from build123d import *

# Parameters (mm, degrees)
SKETCH1_W           = 100
SKETCH1_H           = 100
SKETCH1_W_2         = 96
SKETCH1_H_2         = 96
EXTRUDE_THIN1_DEPTH = 10
FILLET1_R           = 5
FILLET2_R           = 3
BOSS_EXTRUDE1_DEPTH = 1


with BuildPart() as part:
    # Sketch1 → Extrude-Thin1 (new body)
    with BuildSketch(Plane(origin=(0, 0, 0), x_dir=(1, 0, 0), z_dir=(0, 1, 0))):
        Rectangle(SKETCH1_W, SKETCH1_H)
        Rectangle(SKETCH1_W_2, SKETCH1_H_2, mode=Mode.SUBTRACT)
    extrude(amount=EXTRUDE_THIN1_DEPTH)

    # Fillet1
    fillet1_edges = [part.edges().sort_by_distance(p)[0] for p in [
        (50, 5, 50),
        (-50, 5, 50),
        (-50, 5, -50),
        (50, 5, -50),
    ]]
    fillet(fillet1_edges, radius=FILLET1_R)

    # Fillet2
    fillet2_edges = [part.edges().sort_by_distance(p)[0] for p in [
        (48, 5, 48),
        (48, 5, -48),
        (-48, 5, -48),
        (-48, 5, 48),
    ]]
    fillet(fillet2_edges, radius=FILLET2_R)

    # Sketch2 → Boss-Extrude1 (add)
    with BuildSketch(Plane.XZ):
        with BuildLine():
            Line((45, 50), (-45, 50))
            ThreePointArc((-45, 50), (-48.535533906, 48.535533906), (-50, 45))
            Line((-50, 45), (-50, -45))
            ThreePointArc((-50, -45), (-48.535533906, -48.535533906), (-45, -50))
            Line((-45, -50), (45, -50))
            ThreePointArc((45, -50), (48.535533906, -48.535533906), (50, -45))
            Line((50, -45), (50, 45))
            ThreePointArc((50, 45), (48.535533906, 48.535533906), (45, 50))
        make_face()
    extrude(amount=BOSS_EXTRUDE1_DEPTH)


solid = part.part
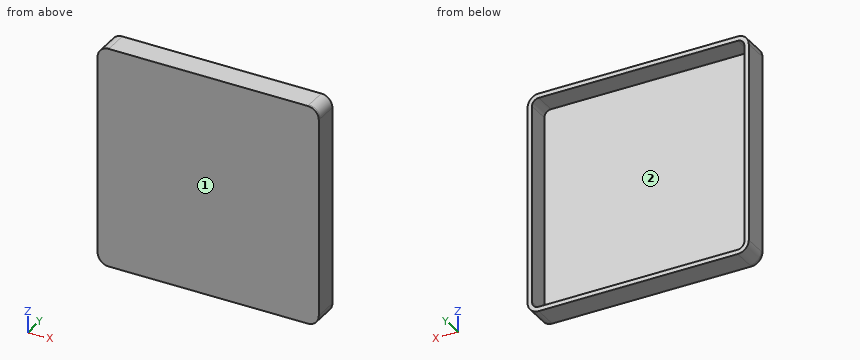
Here's how the part is built. I have some questions about the finished solid (model axes, mm). Face numbers are marked on the shaded views. Coordinates: 2 decimals unless noted, no trailing zeros. Write each loop counter-clockwise with the first axis right and the second up, starting at its lowest first coordinate (ties: lowest second). Pieces come first, ordered by that corner, then holes.
Item 1: If I drill on line 1 (Z direction, x = -40.5, y = 2.25); line 2 (Y direction, x = -7.5, z = -3), over which ranges is the centre line in solid material (lowest first)?
Item 2: I want a section at B-B on x = 34. Write out the boundary of the cut face in (y, z).
Item 3: If we mould it in two halves opening along Z, with no side actions, what happens to the marked faces 1 and 2? For each: +Z half, -Z half, draft (parallel to the pull), parting line (faces both ways), or undercut.
Item 4: I want a section at A-A on y = 2.25. Write out the boundary of the cut face in (x, z), and give its area (3 significant figures).
Item 5: I want a section at C-C on z = 28. Write out the boundary of the cut face in (x, y), and give its area (3 significant figures).
Findings below:
1. line 1: z = -50 to -48, 48 to 50
1. line 2: y = -1 to 0
2. outline: (-1, -50) - (10, -50) - (10, -48) - (0, -48) - (0, 48) - (10, 48) - (10, 50) - (-1, 50) - close
3. face 1: draft
3. face 2: undercut
4. outline: (-50, -45) arc R5 ccw to (-45, -50) - (45, -50) arc R5 ccw to (50, -45) - (50, 45) arc R5 ccw to (45, 50) - (-45, 50) arc R5 ccw to (-50, 45) - close; hole (-48, -45) arc R3 ccw to (-45, -48) - (45, -48) arc R3 ccw to (48, -45) - (48, 45) arc R3 ccw to (45, 48) - (-45, 48) arc R3 ccw to (-48, 45) - close
4. area: 770 mm2
5. outline: (-50, -1) - (50, -1) - (50, 10) - (48, 10) - (48, 0) - (-48, 0) - (-48, 10) - (-50, 10) - close
5. area: 140 mm2
